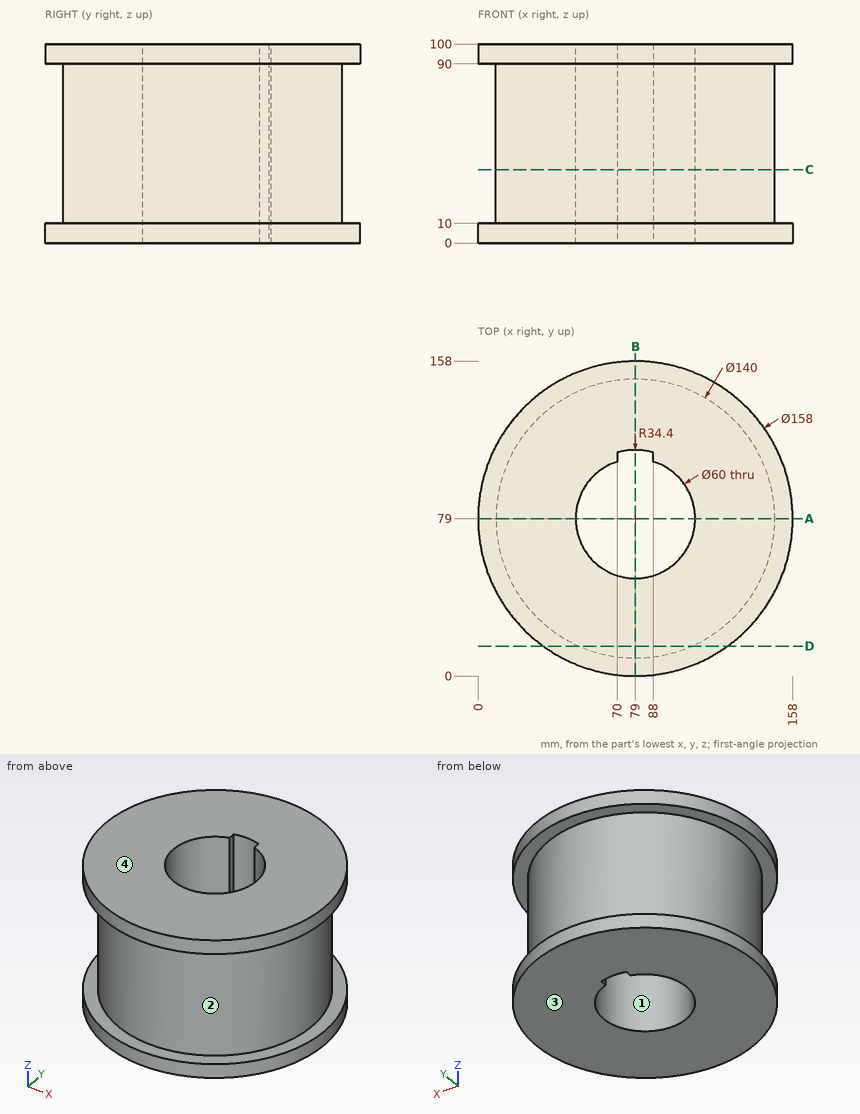
Could you check a few things on this drawing? It's one solid part, dimensions in mm from its lowest x, y, z. Coordinates: 2 decimals unless noted, no trailing zeros. Write each loop counter-clockwise with the first axis right and the second up, starting at its lowest first coordinate (ties: lowest second). Pieces come first, ordered by that corner, then holes.
1) If we section it at C-C (z = 37): List the corners of the cut face in (x, y) for me, plus the area to 3 significant figures.
Filled in:
outline: circle Ø140 at (79, 79); hole (70, 107.62) arc R30 ccw (long way) to (88, 107.62) - (88, 112.2) arc R34.4 ccw to (70, 112.2) - close
area: 12,500 mm2
2) If we section it at A-A (y = 79): List the corners of the cut face in (x, z) for me, plus the area to 3 significant figures.
Filled in:
outline: (0, 0) - (49, 0) - (49, 100) - (0, 100) - (0, 90) - (9, 90) - (9, 10) - (0, 10) - close; (109, 0) - (158, 0) - (158, 10) - (149, 10) - (149, 90) - (158, 90) - (158, 100) - (109, 100) - close
area: 8,360 mm2
3) Thinking about a two-plate mould opening in Z: for the marked faces 1, 2, 3 and 4, which applies, +Z half, -Z half, draft (parallel to the pull), parting line (faces both ways), or undercut?
Filled in:
face 1: draft
face 2: undercut
face 3: -Z half
face 4: +Z half
4) If we section it at D-D (y = 15): List the corners of the cut face in (x, z) for me.
Filled in:
outline: (32.69, 0) - (125.31, 0) - (125.31, 10) - (107.35, 10) - (107.35, 90) - (125.31, 90) - (125.31, 100) - (32.69, 100) - (32.69, 90) - (50.65, 90) - (50.65, 10) - (32.69, 10) - close
5) If we section it at B-B (x = 79): List the corners of the cut face in (y, z) for me.
Filled in:
outline: (0, 0) - (49, 0) - (49, 100) - (0, 100) - (0, 90) - (9, 90) - (9, 10) - (0, 10) - close; (113.4, 0) - (158, 0) - (158, 10) - (149, 10) - (149, 90) - (158, 90) - (158, 100) - (113.4, 100) - close
6) I'm going to push flat-ended pins straight in: pin 1 (5 mm diameter, centred on y = 109, z = 36.5, fed in from +X); pin 2 (6 mm diameter, centred on y = 106.5, z = 89.5, fed in from +X); pin 3 (6 mm diameter, centred on x = 48, z = 28, fed in from -Y). Where does each tip first touch, or does it pass through?
Filled in:
pin 1: stops at x = 143.37
pin 2: stops at x = 154.09
pin 3: stops at y = 14.84
7) If I drill on line 1 (Y direction, x = 79, z = 62); line 2 (Y direction, x = 106, z = 64.5); line 3 (X direction, y = 66, z = 51.5), over which ranges is the centre line in solid material (lowest first)?
Filled in:
line 1: y = 9 to 49, 113.4 to 149
line 2: y = 14.42 to 65.92, 92.08 to 143.58
line 3: x = 10.22 to 51.96, 106.04 to 147.78
